The listing builds one solid part. Answer for the finished solid, in the listing's coordinates (mm). Coordinates: 2 decimals unless noted, no trailing zeros. Write each loop counter-clockwise with the first axis right and the second up, starting at its lowest first coordinate (ties: lowest second). Pieces come first, ordered by that corner, then holes.
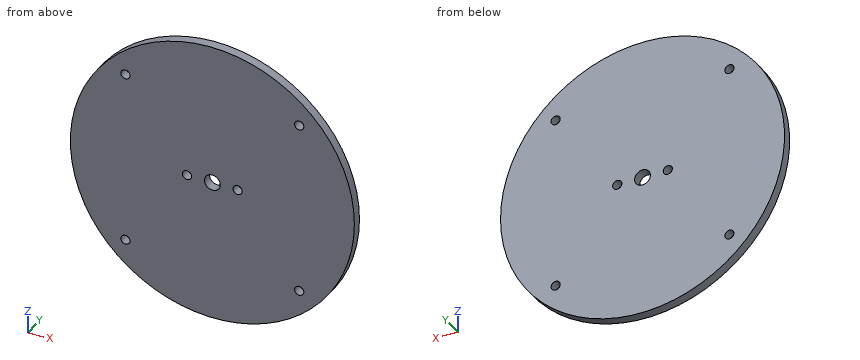
from build123d import *

# Parameters (mm, degrees)
F0_R     = 44.95
F1_DEPTH = 3
F2_R     = 1.45
F2_R_2   = 2.5
F3_DEPTH = 3.001
F4_R     = 1.45
F5_DEPTH = 3.001


with BuildPart() as f1:
    # F0 (on Front) → F1 (new body)
    with BuildSketch(Plane.XZ):
        Circle(F0_R)
    extrude(amount=F1_DEPTH)

    # F2 (on face) → F3 (cut, through all)
    with BuildSketch(Plane.XZ.offset(3)):
        with Locations((-8, 0)):
            Circle(F2_R)
        with Locations((8, 0)):
            Circle(F2_R)
        Circle(F2_R_2)
    extrude(amount=-F3_DEPTH, mode=Mode.SUBTRACT)

    # F4 (on face) → F5 (cut, through all)
    with BuildSketch(Plane.XZ.offset(3)):
        with Locations((-27.5, 27.5)):
            Circle(F4_R)
        with Locations((27.5, 27.5)):
            Circle(F4_R)
        with Locations((-27.5, -27.5)):
            Circle(F4_R)
        with Locations((27.5, -27.5)):
            Circle(F4_R)
    extrude(amount=-F5_DEPTH, mode=Mode.SUBTRACT)


solid = f1.part
1. Find the intervals of material crossed by L1, parallel to Z at x = 27.5, y = -2.4; L2, parallel to Z at x = 0, y = -1.3; L3, parallel to X at y = -0.3, z = 1, in increasing order.
Results found:
L1: z = -35.56 to -28.95, -26.05 to 26.05, 28.95 to 35.56
L2: z = -44.95 to -2.5, 2.5 to 44.95
L3: x = -44.94 to -9.05, -6.95 to -2.29, 2.29 to 6.95, 9.05 to 44.94
2. Section B-B on x = 0 is taken. Give the vertices of the cut face in (y, z), then the cut area to 3 significant figures.
Results found:
outline: (-3, -44.95) - (0, -44.95) - (0, -2.5) - (-3, -2.5) - close; (-3, 2.5) - (0, 2.5) - (0, 44.95) - (-3, 44.95) - close
area: 255 mm2
3. Flat-ended cylindrical pins translate along their axes: P1, Ø2.5, axis at x = 8, z = 0, coming from the +Y side; P2, Ø1, axis at x = -24, y = -0.5, coming from the +Z side. Find the tip coordinate at first contact, or state that the pin passes through.
Results found:
P1: passes through
P2: stops at z = 38.32
4. Section A-A on y = -2.05 is taken. Give the vertices of the cut face in (x, z).
Results found:
outline: circle Ø89.9 at (0, 0); hole circle Ø2.9 at (-27.5, -27.5); hole circle Ø2.9 at (-27.5, 27.5); hole circle Ø2.9 at (-8, 0); hole circle Ø5 at (0, 0); hole circle Ø2.9 at (8, 0); hole circle Ø2.9 at (27.5, -27.5); hole circle Ø2.9 at (27.5, 27.5)
5. Section D-D on x = 27.5 is taken. Give the vertices of the cut face in (y, z), then the cut area to 3 significant figures.
Results found:
outline: (-3, -35.56) - (0, -35.56) - (0, -28.95) - (-3, -28.95) - close; (-3, -26.05) - (0, -26.05) - (0, 26.05) - (-3, 26.05) - close; (-3, 28.95) - (0, 28.95) - (0, 35.56) - (-3, 35.56) - close
area: 196 mm2
6. Section C-C on z = 0 is taken. Give the vertices of the cut face in (x, y), then the cut area to 3 significant figures.
Results found:
outline: (-44.95, -3) - (-9.45, -3) - (-9.45, 0) - (-44.95, 0) - close; (-6.55, -3) - (-2.5, -3) - (-2.5, 0) - (-6.55, 0) - close; (2.5, -3) - (6.55, -3) - (6.55, 0) - (2.5, 0) - close; (9.45, -3) - (44.95, -3) - (44.95, 0) - (9.45, 0) - close
area: 237 mm2
